Autodesk Inventor part; units mm, degrees
ref_plane "YZ Plane" through (0, 0, 0) normal (1, 0, 0) x (0, 1, 0)
ref_plane "XZ Plane" through (0, 0, 0) normal (0, 1, 0) x (-1, 0, 0)
ref_plane "XY Plane" through (0, 0, 0) normal (0, 0, 1) x (1, 0, 0)
sketch "Sketch1" plane through (0, 0, 0) normal (0, 0, 1) x (1, 0, 0)
  line L0 (-10.2957, 5.2289) -> (52.5693, 5.2289)
  line L1 (-10.2957, 5.2289) -> (15.9234, -93.8311) construction
  line L2 (15.9234, -93.8311) -> (26.3501, -93.8311) construction
  line L3 (15.9234, -93.8311) -> (15.9234, -106.5311)
  line L4 (26.3501, -93.8311) -> (26.3501, -106.5311)
  arc A0 (26.3501, -87.7106) -> (26.3501, -93.8311) centre (36.9972, -90.7709) ccw
  arc A1 (26.3501, -87.7106) -> (52.5693, 5.2289) centre (-125.2627, 5.2289) ccw
  line L5 (21.1368, 5.2289) -> (21.1368, -93.8311) construction
  arc A2 (15.9234, -93.8311) -> (15.9234, -87.7106) centre (5.2764, -90.7709) ccw
  arc A3 (-10.2957, 5.2289) -> (15.9234, -87.7106) centre (167.5363, 5.2289) ccw
  line L6 (26.3501, -106.5311) -> (23.352, -113.2427) construction
  line L7 (26.3501, -106.5311) -> (22.8287, -111.1925)
  line L8 (22.8287, -111.1925) -> (19.4449, -111.1925)
  line L9 (15.9234, -106.5311) -> (19.4449, -111.1925)
  point P0 (0, 0)
  point P1 (8.355, -65.2363)
  dimension "d10" = 10.4267
  dimension "d11" = 12.7
  dimension "d12" = 99.06
  dimension "d15" = 5.842
  dimension "d16" = 5.842
  dimension "d19" = 62.865
  dimension "d20" = 3.3838
extrude "Extrusion1" add sketch "Sketch1" along normal blind 0.7112
sketch "Sketch2" plane through (0, 0, 0.7112) normal (0, 0, 1) x (1, 0, 0)
  arc A0 (-10.2957, 5.2289) -> (15.9234, -87.7106) centre (167.5363, 5.2289) ccw
  arc A1 (26.3501, -87.7106) -> (26.3501, -93.8311) centre (36.9972, -90.7709) ccw
  arc A2 (15.9234, -93.8311) -> (15.9234, -87.7106) centre (5.2764, -90.7709) ccw
  line L0 (15.9234, -87.7106) -> (26.3501, -87.7106)
  point P0 (0, 0)
sketch "Sketch3" plane through (0, 0, 0.7112) normal (0, 0, 1) x (1, 0, 0)
  arc A0 (-10.2957, 5.2289) -> (15.9234, -87.7106) centre (167.5363, 5.2289) ccw
  line L0 (8.288, -73.9178) -> (33.9856, -73.9178)
  arc A1 (26.3501, -87.7106) -> (52.5693, 5.2289) centre (-125.2627, 5.2289) ccw
  point P0 (0, 0)
properties part number "Dis"
Geometry check sheet. Reference: the model listing, model coordinates, mm. Give positions to 0.01 mm unless a question says otherwise; leave off trailing zeros. Loops run counter-clockwise (first coordinate to the right, second up) from the corner with the lowest first, then second, coordinate; pieces in that order, holes last. Notation, with made-up numbers: (86.25, -39.75) -> (111.25, -39.75) arc R33 ccw to (111.25, -6.75) -> close; hole circle Ø10 at (29.5, 78). An arc over 180 degrees is marked (long way). Answer in a Markdown table with one row per item. Add a question column.
1) Cross-section at B-B on x = 34.5. Record the boundary of the cut face in (y, z), and give its area (3 significant figures).
2) Cross-section at A-A on z = 0.4. Record the boundary of the cut face in (x, y), and give its area (3 significant figures).
3) Cross-section at C-C on y = -99.5. Record the boundary of the cut face in (x, z).
4) Material ranges on probe 1 along X at (y, z) = (-91, 0.5); probe 2 along X at (y, z) = (-28.5, 0.45); probe 3 along Y at (x, z) = (32, 0.25), recorded low to high. Write a range as from..to.
Outcome:
| question | item | result |
|---|---|---|
| 1 | outline | (-72.87, 0) -> (5.23, 0) -> (5.23, 0.71) -> (-72.87, 0.71) -> close |
| 1 | area | 55.5 mm^2 |
| 2 | outline | (-10.3, 5.23) arc R177.83 ccw to (15.92, -87.71) arc R11.08 cw to (15.92, -93.83) -> (15.92, -106.53) -> (19.44, -111.19) -> (22.83, -111.19) -> (26.35, -106.53) -> (26.35, -93.83) arc R11.08 cw to (26.35, -87.71) arc R177.83 ccw to (52.57, 5.23) -> close |
| 2 | area | 4,490 mm^2 |
| 3 | outline | (15.92, 0) -> (26.35, 0) -> (26.35, 0.71) -> (15.92, 0.71) -> close |
| 4 | probe 1 | x = 16.35..25.92 |
| 4 | probe 2 | x = -7.07..49.34 |
| 4 | probe 3 | y = -77.79..5.23 |
